Could you check a few things on this model? Use its own coordinates, in mm. Face numbers are marked on the shaded views. A direction names the side the tool comes from. Give positions to 0.01 mm unless a question says otherwise; leave off trailing zeros. Write each loop counter-clockwise with the first axis right and the second up, starting at its lowest first coordinate (ties: lowest second). Pieces come first, ordered by that corner, then holes. Notation, with made-up numbers: (-2.5, 29) - (2.5, 29) arc R8 ccw to (2.5, 41) - close; hole circle Ø6 at (42.25, 70.5). An arc over 180 degrees is marked (long way). Answer as a JSON object with one key per item and string values. Group by question number.
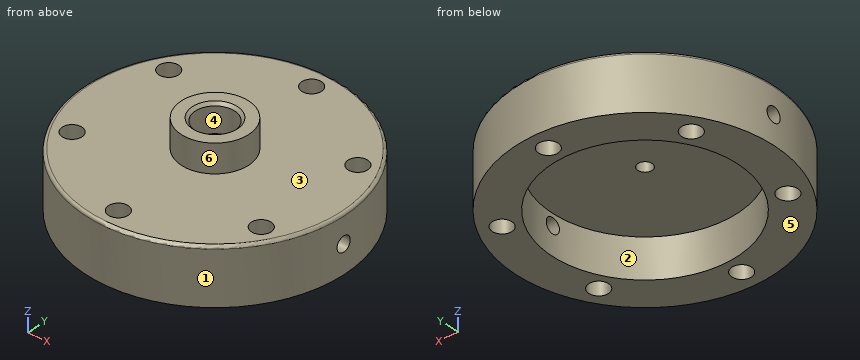
```python
from build123d import *

# Parameters (mm, degrees)
SKETCH2_R               = 46
SKETCH2_R_2             = 3.5
SKETCH2_R_3             = 2.5
BOSS_EXTRUDE1_DEPTH     = 20
SKETCH3_R               = 12
SKETCH3_R_2             = 7
BOSS_EXTRUDE2_DEPTH     = 10
CHAMFER1_SIZE           = 1
SKETCH6_R               = 33
CUT_EXTRUDE1_DEPTH      = 14
FILLET1_R               = 1
SKETCH7_R               = 2.66023902
CUT_EXTRUDE2_DEPTH      = 47
CUT_EXTRUDE2_DEPTH_BACK = 47


with BuildPart() as part:
    # Sketch2 → Boss-Extrude1 (new body)
    with BuildSketch(Plane.XY):
        Circle(SKETCH2_R)
        with Locations((0, 39)):
            Circle(SKETCH2_R_2, mode=Mode.SUBTRACT)
        Circle(SKETCH2_R_3, mode=Mode.SUBTRACT)
        with Locations((33.774990748, 19.5)):
            Circle(SKETCH2_R_2, mode=Mode.SUBTRACT)
        with Locations((33.774990748, -19.5)):
            Circle(SKETCH2_R_2, mode=Mode.SUBTRACT)
        with Locations((0, -39)):
            Circle(SKETCH2_R_2, mode=Mode.SUBTRACT)
        with Locations((-33.774990748, -19.5)):
            Circle(SKETCH2_R_2, mode=Mode.SUBTRACT)
        with Locations((-33.774990748, 19.5)):
            Circle(SKETCH2_R_2, mode=Mode.SUBTRACT)
    extrude(amount=BOSS_EXTRUDE1_DEPTH)

    # Sketch3 → Boss-Extrude2 (add)
    with BuildSketch(Plane.XY.offset(20)):
        Circle(SKETCH3_R)
        Circle(SKETCH3_R_2, mode=Mode.SUBTRACT)
    extrude(amount=BOSS_EXTRUDE2_DEPTH)

    # Chamfer1
    chamfer1_edges = [part.edges().sort_by_distance(p)[0] for p in [
        (-7, 0, 30),
    ]]
    chamfer(chamfer1_edges, length=CHAMFER1_SIZE)

    # Sketch6 → Cut-Extrude1 (cut)
    with BuildSketch(Plane(origin=(0, 0, 0), x_dir=(-1, 0, 0), z_dir=(0, 0, -1))):
        Circle(SKETCH6_R)
    extrude(amount=-CUT_EXTRUDE1_DEPTH, mode=Mode.SUBTRACT)

    # Fillet1
    fillet1_edges = [part.edges().sort_by_distance(p)[0] for p in [
        (-46, 0, 20),
    ]]
    fillet(fillet1_edges, radius=FILLET1_R)

    # Sketch7 → Cut-Extrude2 (cut, two sides)
    with BuildSketch(Plane(origin=(0, 0, 0), x_dir=(0, 0, -1), z_dir=(1, 0, 0))) as cut_extrude2_sk:
        with Locations((-10, 0)):
            Circle(SKETCH7_R)
    extrude(amount=CUT_EXTRUDE2_DEPTH, mode=Mode.SUBTRACT)
    extrude(cut_extrude2_sk.sketch, amount=-CUT_EXTRUDE2_DEPTH_BACK, mode=Mode.SUBTRACT)


solid = part.part
```
(1) I want a section at B-B, the plane z = 2. Please give me the cut outline in (x, y) (3 decimals), and give its area (3 significant figures).
(2) If we mould it in two halves opening along Y, with no side actions, what happens to the marked faces 4, 5 and 6? For each: +Y half, -Y half, draft (parallel to the pull), parting line (faces both ways), or undercut.
(3) I want a section at A-A, the plane z = 9.5. Please give me the cut outline in (x, y) (3 decimals), and give its area (3 significant figures).
(4) Will these pins go through, and if not, where does the flat tip stop? P1, Ø6.5, axis at x = 0, y = 0, coming from the -Z side; P2, Ø9, axis at x = -33.77, y = -19.5, coming from the +Z side; P3, Ø8, axis at x = -33.77, y = 19.5, coming from the -Z side; P4, Ø12, axis at y = -14.5, z = 21.5, coming from the +X side.
(5) I want a section at C-C, the plane y = 19.5. State how many separate pieces and enclosed holes the cut face has, and give its area (3 significant figures).
(6) I need wall thicknesses on L1, parallel to Y at x = 0, z = 8.75; L2, parallel to X at y = -21, z = 12; L3, parallel to X at y = 0.5, z = 28. Which ranges of each line are inside material? Lowest first, please.
(7) I want a section at D-D, the plane z = 26. Please give me the cut outline in (x, y), and give its area (3 significant figures).
(8) For the marked faces 1, 2 and 3, which set-ups out of +Z, -Z, +X, -X, +Y, -Y let a thin tool reach every point of the face, with its end or its side?
Entries:
{
 "1": {"outline": "circle Ø92 at (0, 0); hole circle Ø7 at (-33.775, -19.5); hole circle Ø7 at (-33.775, 19.5); hole circle Ø66 at (0, 0); hole circle Ø7 at (0, -39); hole circle Ø7 at (0, 39); hole circle Ø7 at (33.775, -19.5); hole circle Ø7 at (33.775, 19.5)", "area": "3,000 mm^2"},
 "2": {"face 4": "undercut", "face 5": "draft", "face 6": "parting line"},
 "3": {"outline": "(-45.926, -2.613) arc R46 ccw to (45.926, -2.613) - (32.896, -2.613) arc R33 cw to (-32.896, -2.613) - close; (-45.926, 2.613) - (-32.896, 2.613) arc R33 cw to (32.896, 2.613) - (45.926, 2.613) arc R46 ccw to start; hole circle Ø7 at (-33.775, -19.5); hole circle Ø7 at (-33.775, 19.5); hole circle Ø7 at (0, -39); hole circle Ø7 at (0, 39); hole circle Ø7 at (33.775, -19.5); hole circle Ø7 at (33.775, 19.5)", "area": "2,860 mm^2"},
 "4": {"P1": "z = 14", "P2": "z = 20", "P3": "z = 0", "P4": "x = 45.11"},
 "5": {"separate pieces": "3", "enclosed holes": "0", "area": "641 mm^2"},
 "6": {"L1": "-46 to -42.5, -35.5 to -33, 33 to 35.5, 42.5 to 46", "L2": "-40.93 to -36.94, -30.61 to -25.46, 25.46 to 30.61, 36.94 to 40.93", "L3": "-11.99 to -6.98, 6.98 to 11.99"},
 "7": {"outline": "circle Ø24 at (0, 0); hole circle Ø14 at (0, 0)", "area": "298 mm^2"},
 "8": {"face 1": "+Z, -Z", "face 2": "-Z", "face 3": "+Z"}
}
